The figure shows three views and two pictorial views of one solid part (mm, origin at its lowest corner). Answer the questions. Coordinates: 2 decimals unless noted, no trailing zeros. Write each loop counter-clockwise with the first axis right and the second up, starting at its lowest first coordinate (ties: lowest second). Pieces come first, ordered by that corner, then holes. Notation, with made-up numbers: M -19,24.25 L 37,24.25 A4 cw 37,31.25 Z; hole C 8,13 d4. An arc over 180 degrees is marked long. Use a Markdown table: item, result. Add a question column.
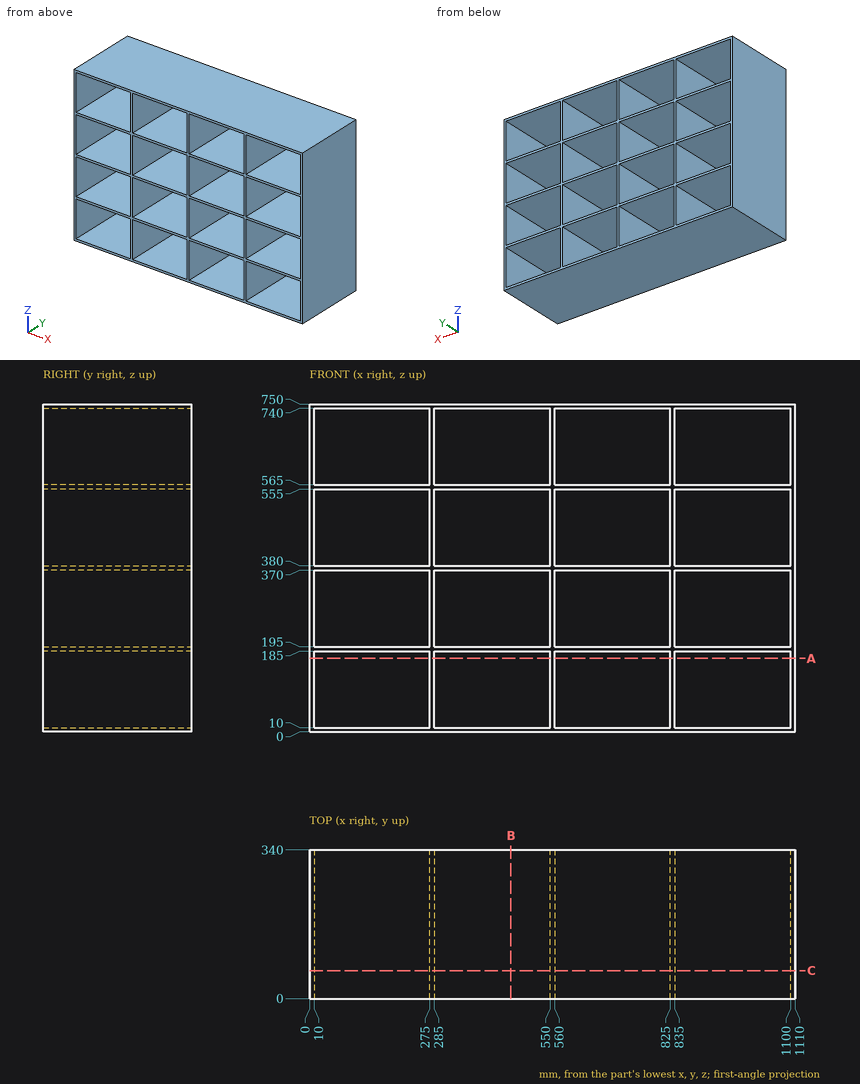
Item 1: Find section A-A on z = 168. Give the vertices of the cut face in (x, y).
Item 2: Find section B-B on x = 460. Give the vertices of the cut face in (y, z), then the cut area to 3 significant figures.
Item 3: Find section C-C on y = 64. Count the separate pieces of the cut face and the enclosed holes in it, then the cut area to 3 significant figures.
Item 4: This flat-tipped pin is pushed along its axis until it touches: pin 1 (8 mm diameter, centred on x = 672, y = 35.5, fed in from -Z). Where does it stop, or does it pass through?
Item 5: Consider probe 1 along Z at (x, y) = (327.5, 155.5); probe 2 along X at (y, z) = (84, 70.5). Determine where each line is inside the solid, lowest interval first.
Geometry says:
| question | item | result |
|---|---|---|
| 1 | outline | M 0,0 L 10,0 L 10,340 L 0,340 Z; M 275,0 L 285,0 L 285,340 L 275,340 Z; M 550,0 L 560,0 L 560,340 L 550,340 Z; M 825,0 L 835,0 L 835,340 L 825,340 Z; M 1100,0 L 1110,0 L 1110,340 L 1100,340 Z |
| 2 | outline | M 0,0 L 340,0 L 340,10 L 0,10 Z; M 0,185 L 340,185 L 340,195 L 0,195 Z; M 0,370 L 340,370 L 340,380 L 0,380 Z; M 0,555 L 340,555 L 340,565 L 0,565 Z; M 0,740 L 340,740 L 340,750 L 0,750 Z |
| 2 | area | 17,000 mm2 |
| 3 | separate pieces | 1 |
| 3 | enclosed holes | 16 |
| 3 | area | 90,500 mm2 |
| 4 | pin 1 | stops at z = 0 |
| 5 | probe 1 | z = 0 to 10, 185 to 195, 370 to 380, 555 to 565, 740 to 750 |
| 5 | probe 2 | x = 0 to 10, 275 to 285, 550 to 560, 825 to 835, 1100 to 1110 |
